Here's how the part is built. I have some questions about the finished solid (model axes, mm). Face numbers are marked on the shaded views. Give positions to 0.01 mm unless a question says otherwise; leave off trailing zeros. Loops run counter-clockwise (first coordinate to the right, second up) from the corner with the lowest first, then second, coordinate; pieces in that order, holes last. Notation, with made-up numbers: M -29.5,-35 L -23.5,-35 A15 ccw -23.5,-9 Z; hole C 50.5,-3.5 d2. An arc over 180 degrees is marked long. Write item = value, one per line. Start each with the question number.
```python
from build123d import *

# Parameters (mm, degrees)
SKETCH_1_R           = 36
SKETCH_1_R_2         = 25
EXTRUDE_1_DEPTH      = 3
EXTRUDE_START        = 1
SKETCH_3_R           = 36
SKETCH_3_R_2         = 35
EXTRUDE_2_DEPTH      = 1
HOLE_WIZARD_M2_5_1_D = 2.5


with BuildPart() as part:
    # 草图1 → 凸台-拉伸1 (new body)
    with BuildSketch(Plane(origin=(0, 0, 0), x_dir=(1, 0, 0), z_dir=(0, 1, 0))):
        with Locations(Location((0, 0, 0), (0, 0, 270))):
            Circle(SKETCH_1_R)
        with Locations(Location((0, 0, 0), (0, 0, 270))):
            Circle(SKETCH_1_R_2, mode=Mode.SUBTRACT)
    extrude(amount=EXTRUDE_1_DEPTH)

    # 草图3 → 凸台-拉伸2 (add)
    with BuildSketch(Plane.XZ.offset(EXTRUDE_START)):
        with Locations(Location((0, 0, 0), (0, 0, 270))):
            Circle(SKETCH_3_R)
        with Locations(Location((0, 0, 0), (0, 0, 270))):
            Circle(SKETCH_3_R_2, mode=Mode.SUBTRACT)
    extrude(amount=-EXTRUDE_2_DEPTH)

    # M2.5 螺纹孔1 (through all)
    with Locations(Plane(origin=(0, 0, 32.5), x_dir=(0, 0, -1), z_dir=(0, -1, 0))):
        with Locations((0, 0), (16.25, 28.145825623), (48.75, 28.145825623), (16.25, -28.145825623), (48.75, -28.145825623), (65, 0)):
            Hole(HOLE_WIZARD_M2_5_1_D / 2)


solid = part.part
```
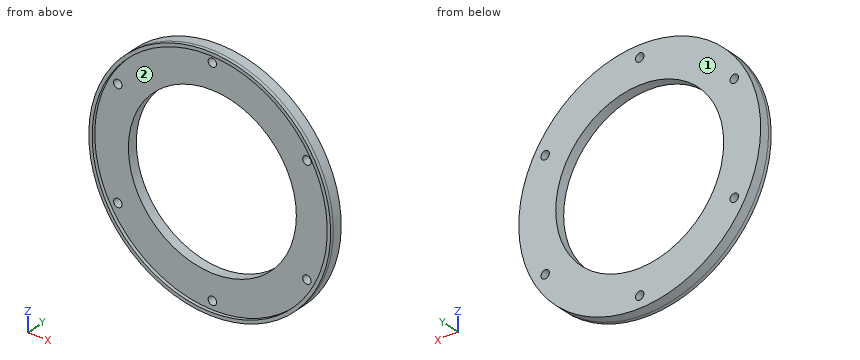
Q1. Will these pins go through, and if not, where does the flat tip stop? pin 1 (12 mm diameter, centred on x = -8.5, z = -26.5, fed in from -Y); pin 2 (2 mm diameter, centred on y = 2.5, z = 3, fed in from -X).
Q2. We'd pull the mould along X, two halves only. Please class the marked faces 1 and 2: pulls with the +X half, pulls with the -X half, needs draft (parallel to the pull), parting line crosses it, or undercut.
Q3. If we section it at C-C, the plane x = -14.5: List the corners of the cut face in (y, z) for me, then the cut area to 3 significant figures.
Q4. If we section it at B-B, the plane z = 0: List the corners of the cut face in (x, y) for me, then the cut area to 3 significant figures.
Q5. If we section it at D-D, the plane z = 16.25: List the corners of the cut face in (x, y) for me.
Q6. If I drill on line 1 along Z through (x, y) = (-29, 2.75); line 2 along Z through (x, y) = (-27.5, 1.55); line 3 along Y through (x, z) = (22, 25), over which ranges is the centre line in solid material (lowest first)?
Q7. If we section it at A-A, the plane x = 0: List the corners of the cut face in (y, z) for me, then the cut area to 3 significant figures.
Resolved:
q1.pin_1 = 0
q1.pin_2 = -35.94
q2.face_1 = needs draft
q2.face_2 = undercut
q3.outline = M -1,-32.95 L 3,-32.95 L 3,-20.37 L 0,-20.37 L 0,-31.86 L -1,-31.86 Z; M -1,31.86 L 0,31.86 L 0,20.37 L 3,20.37 L 3,32.95 L -1,32.95 Z
q3.area = 77.7 mm²
q4.outline = M -36,-1 L -35,-1 L -35,0 L -25,0 L -25,3 L -36,3 Z; M 25,0 L 35,0 L 35,-1 L 36,-1 L 36,3 L 25,3 Z
q4.area = 68.0 mm²
q5.outline = M -32.12,-1 L -31,-1 L -31,0 L -29.4,0 L -29.4,3 L -32.12,3 Z; M -26.9,0 L -19,0 L -19,3 L -26.9,3 Z; M 19,0 L 26.9,0 L 26.9,3 L 19,3 Z; M 29.4,0 L 31,0 L 31,-1 L 32.12,-1 L 32.12,3 L 29.4,3 Z
q6.line_1 = -21.33 to -17.16, -15.34 to 15.34, 17.16 to 21.33
q6.line_2 = -23.23 to -17.32, -15.18 to 15.18, 17.32 to 23.23
q6.line_3 = 0 to 3
q7.outline = M -1,-36 L 3,-36 L 3,-33.75 L 0,-33.75 L 0,-35 L -1,-35 Z; M -1,35 L 0,35 L 0,33.75 L 3,33.75 L 3,36 L -1,36 Z; M 0,-31.25 L 3,-31.25 L 3,-25 L 0,-25 Z; M 0,25 L 3,25 L 3,31.25 L 0,31.25 Z
q7.area = 53.0 mm²
